Could you check a few things on this drawing? It's one solid part, dimensions in mm from its lowest x, y, z. A direction names the side the tool comes from. Give positions to 0.01 mm unless a question says otherwise; leave off trailing zeros. Loops run counter-clockwise (first coordinate to the right, second up) from the corner with the lowest first, then second, coordinate; pieces in that order, holes last. Notation, with made-up numbers: (-36, 18.5) - (-29, 18.5) arc R20 ccw to (-29, 52.5) - close; hole circle Ø7 at (53, 45.5). An arc over 180 degrees is marked (long way). Return JSON: item names as keys, results as strings. Group by question number.
(1) If we section it at D-D (z = 7.25): Please give me the cut outline in (x, y).
(2) On a 3-axis mill with a long thin cutter (end or side, diameter ignored), from which of +Z, -Z, +X, -X, +Y, -Y can I reach the whole of each face in a straight line? I mean the marked faces 1, 2 and 3. Say none if no direction works.
(3) For P1, Ø0.8, axis at x = 6, y = 2, coming from the -Z side; P2, Ø3, axis at x = 2.5, z = 12, coming from the +Y side; P3, Ø0.8, axis at y = 2, z = 10.5, coming from the -X side, each with a flat end and sliding along its axis, tell me the tip position at first contact or that it passes through.
(4) If we section it at C-C (x = 7): Please give me the cut outline in (y, z).
(5) If we section it at B-B (z = 1.75): Please give me the cut outline in (x, y).
(6) If we section it at A-A (y = 1.35): Please give me the cut outline in (x, z), then the cut area to 3 significant figures.
(7) I need wall thicknesses on probe 1 along X at (y, z) = (0.3, 1.75); probe 2 along Z at (x, y) = (9, 0.7); probe 3 along Z at (x, y) = (1.25, 1.05). Which ranges of each line are inside material? Lowest first, please. Write a range as [from, to].
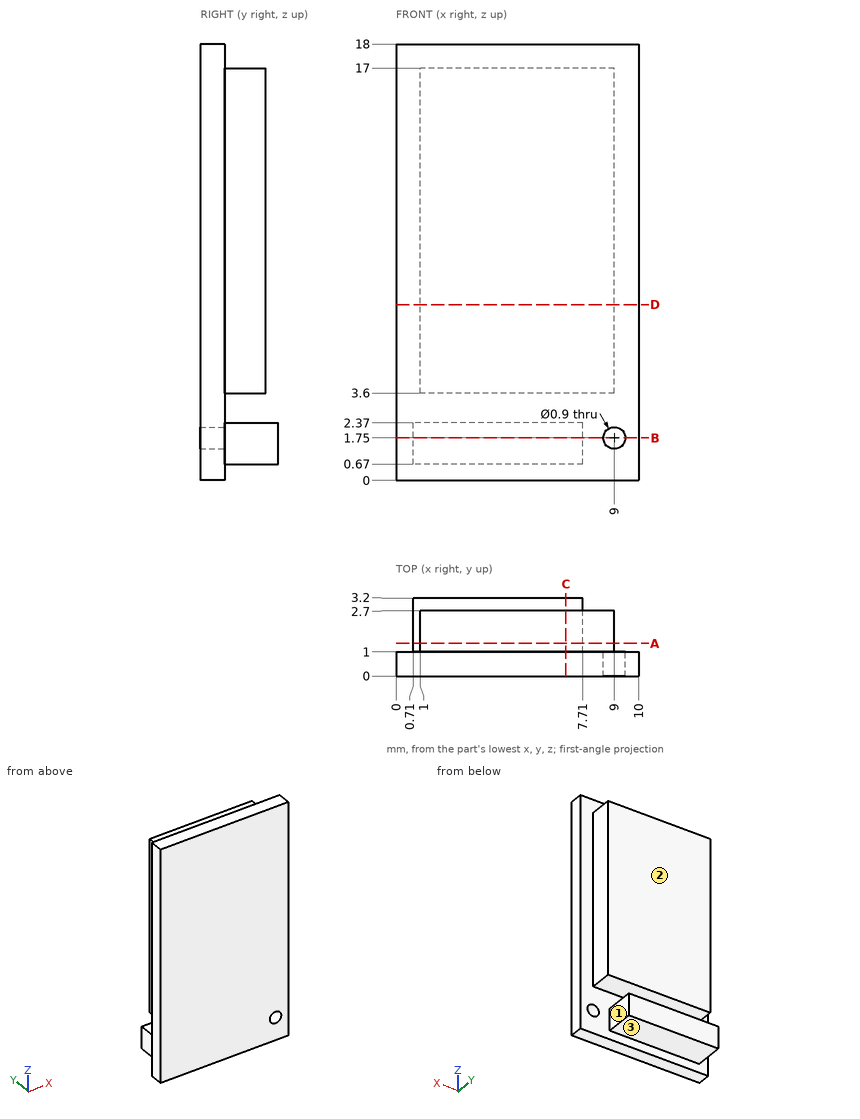
Values:
{
 "1": {"outline": "(0, 0) - (10, 0) - (10, 1) - (9, 1) - (9, 2.7) - (1, 2.7) - (1, 1) - (0, 1) - close"},
 "2": {"face 1": "-Z, +X, +Y", "face 2": "+Z, +X, -X, +Y", "face 3": "-Z, +X, -X, +Y"},
 "3": {"P1": "z = 0.67", "P2": "y = 2.7", "P3": "x = 1"},
 "4": {"outline": "(0, 0) - (1, 0) - (1, 0.67) - (3.2, 0.67) - (3.2, 2.37) - (1, 2.37) - (1, 3.6) - (2.7, 3.6) - (2.7, 17) - (1, 17) - (1, 18) - (0, 18) - close"},
 "5": {"outline": "(0, 0) - (8.55, 0) - (8.55, 1) - (7.71, 1) - (7.71, 3.2) - (0.71, 3.2) - (0.71, 1) - (0, 1) - close; (9.45, 0) - (10, 0) - (10, 1) - (9.45, 1) - close"},
 "6": {"outline": "(0.71, 0.67) - (7.71, 0.67) - (7.71, 2.37) - (0.71, 2.37) - close; (1, 3.6) - (9, 3.6) - (9, 17) - (1, 17) - close", "area": "119 mm2"},
 "7": {"probe 1": "[0, 8.55], [9.45, 10]", "probe 2": "[0, 1.3], [2.2, 18]", "probe 3": "[0.67, 2.37], [3.6, 17]"}
}
